Part model, mm, in its own coordinate system. A direction names the side the tool comes from. Give positions to 0.01 mm unless a question says otherwise; leave off trailing zeros. Write each loop counter-clockwise with the first axis right and the second up, starting at its lowest first coordinate (ties: lowest second). Pieces come first, ordered by that corner, then holes. Notation, with made-up numbers: M -34,15.25 L -19,15.25 A17 cw -19,25.25 Z; hole C -23,31 d3. An arc over 180 degrees is marked long. Answer as CSV lines item,"result". Start each with the question number.
1) Tool access for faces 1 (the flat face through (-3, 10, -14.25)), 2 (the cylindrical face through (33.48, 9.6, -12.43)), 3 (the flat face through (-11, 18, -9)): list every direction of +Z, -Z, +X, -X, +Y, -Y with a clear straight run to the whole face (end or side of a thin tool).
2) Mould opens along Z. For faces 4 (the cylindrical face through (33.48, 9.6, 12.43)), 5 (the flat face through (35, 7, 0)), 6 (the flat face through (0, 9, -17.25)) say: pulls with the +Z half, pulls with the -Z half, needs draft (parallel to the pull), parting line crosses it, or undercut.
3) Slice it at A-A, the plane y = 4.5. Give the cut face in (x, z), plus the area to 3 significant figures.
4) Slice it at C-C, the plane y = 15.5. Give the cut face in (x, z), plus the area to 3 significant figures.
5) Slice it at D-D, the plane x = 7. Give the cut face in (y, z), plus the area to 4 significant figures.
6) Slice it at B-B, the plane x = -24. Give the cut face in (y, z).
7) Pin check, flat tips, straight feed: pin 1 Ø1.6 at (x, z) = (-16.5, 10.5) entering from +Y; pin 2 Ø7 at (x, z) = (18.5, 7) entering from +Y. Stop position of each tip, or through.
8) Wall check: line 1 along X through (y, z) = (3.75, 8); line 2 along Z through (x, y) = (17.5, 10); line 3 along X through (y, z) = (14.75, -7). Give the ranges that are in metal, low to high. Write a range as from..to.
```python
from build123d import *

# Parameters (mm, degrees)
SKETCH1_W           = 70
SKETCH1_H           = 34.5
BOSS_EXTRUDE1_DEPTH = 3
SKETCH2_W           = 70
SKETCH2_H           = 34.5
SKETCH2_W_2         = 64
SKETCH2_H_2         = 28.5
EXTRUDE_THIN1_DEPTH = 15
CUT_EXTRUDE1_REACH  = 76.307
SKETCH3_W           = 26
SKETCH3_H           = 5
SKETCH6_W           = 5
SKETCH6_H           = 28.5
BOSS_EXTRUDE2_DEPTH = 15
SKETCH7_W           = 24
SKETCH7_H           = 8.5
BOSS_EXTRUDE3_DEPTH = 15
SKETCH8_W           = 36.5
SKETCH8_H           = 5.5
BOSS_EXTRUDE4_DEPTH = 13.45
FILLET1_R           = 2
FILLET2_R           = 2
CUT_EXTRUDE6_REACH  = 44.972
SKETCH12_W          = 5
SKETCH12_H          = 23.5
SKETCH13_R          = 1.25
CUT_EXTRUDE7_DEPTH  = 10
FILLET4_R           = 2


with BuildPart() as part:
    # Sketch1 → Boss-Extrude1 (new body)
    with BuildSketch(Plane(origin=(0, 0, 0), x_dir=(1, 0, 0), z_dir=(0, 1, 0))):
        Rectangle(SKETCH1_W, SKETCH1_H)
    extrude(amount=BOSS_EXTRUDE1_DEPTH)

    # Sketch2 → Extrude-Thin1 (add)
    with BuildSketch(Plane(origin=(0, 3, 0), x_dir=(1, 0, 0), z_dir=(0, 1, 0))):
        Rectangle(SKETCH2_W, SKETCH2_H)
        Rectangle(SKETCH2_W_2, SKETCH2_H_2, mode=Mode.SUBTRACT)
    extrude(amount=EXTRUDE_THIN1_DEPTH)

    # Sketch3 → Cut-Extrude1 (cut, up to next)
    with BuildSketch(Plane(origin=(35, 0, 0), x_dir=(0, 0, -1), z_dir=(1, 0, 0)), mode=Mode.PRIVATE) as cut_extrude1_sk1:
        with Locations((0, 11.5)):
            Rectangle(SKETCH3_W, SKETCH3_H)
    cut_extrude1_tool1 = extrude(cut_extrude1_sk1.sketch, amount=-CUT_EXTRUDE1_REACH, mode=Mode.PRIVATE) & part.part
    add(cut_extrude1_tool1.solids().sort_by_distance((35, 11.5, 0))[0], mode=Mode.SUBTRACT)

    # Sketch6 → Boss-Extrude2 (add)
    with BuildSketch(Plane(origin=(0, 3, 0), x_dir=(1, 0, 0), z_dir=(0, 1, 0))):
        with Locations((7, 0)):
            Rectangle(SKETCH6_W, SKETCH6_H)
    extrude(amount=BOSS_EXTRUDE2_DEPTH)

    # Sketch7 → Boss-Extrude3 (add)
    with BuildSketch(Plane(origin=(0, 3, 0), x_dir=(1, 0, 0), z_dir=(0, 1, 0))):
        with Locations((-20, 10)):
            Rectangle(SKETCH7_W, SKETCH7_H)
    extrude(amount=BOSS_EXTRUDE3_DEPTH)

    # Sketch8 → Boss-Extrude4 (add)
    with BuildSketch(Plane(origin=(0, 3, 0), x_dir=(1, 0, 0), z_dir=(0, 1, 0))):
        with Locations((-13.75, -11.5)):
            Rectangle(SKETCH8_W, SKETCH8_H)
    extrude(amount=BOSS_EXTRUDE4_DEPTH)

    # Fillet1
    fillet1_edges = [part.edges().sort_by_distance(p)[0] for p in [
        (33.5, 9, 13),
        (33.5, 14, 13),
        (33.5, 14, -13),
        (33.5, 9, -13),
    ]]
    fillet(fillet1_edges, radius=FILLET1_R)

    # Fillet2
    fillet2_edges = [part.edges().sort_by_distance(p)[0] for p in [
        (35, 9, 17.25),
        (-35, 9, 17.25),
        (-35, 9, -17.25),
        (35, 9, -17.25),
    ]]
    fillet(fillet2_edges, radius=FILLET2_R)

    # Cut-Extrude6: up to this face of the body (flat: up to its plane)
    cut_extrude6_end = Plane(part.part.faces().sort_by_distance((33.5, 9, 0))[0])
    # Sketch12 → Cut-Extrude6 (cut, up to the picked face)
    with BuildSketch(Plane(origin=(0, 18, 0), x_dir=(1, 0, 0), z_dir=(0, 1, 0)), mode=Mode.PRIVATE) as cut_extrude6_sk1:
        with Locations((7, 0)):
            Rectangle(SKETCH12_W, SKETCH12_H)
    cut_extrude6_tool1 = split(extrude(cut_extrude6_sk1.sketch, amount=-CUT_EXTRUDE6_REACH, mode=Mode.PRIVATE), bisect_by=cut_extrude6_end, keep=Keep.BOTH, mode=Mode.PRIVATE)
    add(cut_extrude6_tool1.solids().sort_by(Axis((7, 18, 0), (0, -1, 0)))[0], mode=Mode.SUBTRACT)

    # Sketch13 → Cut-Extrude7 (cut)
    with BuildSketch(Plane(origin=(0, 18, 0), x_dir=(1, 0, 0), z_dir=(0, 1, 0))):
        with Locations(Location((7, 14.25, 0), (0, 0, 270))):
            Circle(SKETCH13_R)
        with Locations(Location((7, -14.25, 0), (0, 0, 90))):
            Circle(SKETCH13_R)
    extrude(amount=-CUT_EXTRUDE7_DEPTH, mode=Mode.SUBTRACT)

    # Fillet4
    fillet4_edges = [part.edges().sort_by_distance(p)[0] for p in [
        (4.5, 10.5, -14.25),
    ]]
    fillet(fillet4_edges, radius=FILLET4_R)


solid = part.part
```
Found:
1,face 1,"+Y"
1,face 2,"+X"
1,face 3,"+Z, -Z, +X, -X, +Y"
2,face 4,"undercut"
2,face 5,"needs draft"
2,face 6,"pulls with the -Z half"
3,outline,"M -35,-15.25 A2 ccw -33,-17.25 L 33,-17.25 A2 ccw 35,-15.25 L 35,15.25 A2 ccw 33,17.25 L -33,17.25 A2 ccw -35,15.25 Z; hole M -32,-5.75 L -8,-5.75 L -8,-14.25 L 2.5,-14.25 A2 ccw 4.5,-12.25 L 4.5,8.75 L -32,8.75 Z; hole M 9.5,-14.25 L 32,-14.25 L 32,14.25 L 9.5,14.25 Z"
3,area,"1,140 mm²"
4,outline,"M -35,-15.25 A2 ccw -33,-17.25 L 33,-17.25 A2 ccw 35,-15.25 L 35,15.25 A2 ccw 33,17.25 L -33,17.25 A2 ccw -35,15.25 Z; hole M -32,-5.75 L -8,-5.75 L -8,-14.25 L 2.5,-14.25 A2 ccw 4.5,-12.25 L 4.5,-11.75 L 9.5,-11.75 L 9.5,-14.25 L 32,-14.25 L 32,14.25 L 9.5,14.25 L 9.5,11.75 L 4.5,11.75 L 4.5,8.75 L -32,8.75 Z; hole C 7,-14.25 d2.5; hole C 7,14.25 d2.5"
4,area,"1,010 mm²"
5,outline,"M 0,-17.25 L 18,-17.25 L 18,-15.5 L 8,-15.5 L 8,-13 L 18,-13 L 18,-11.75 L 9,-11.75 L 9,11.75 L 18,11.75 L 18,13 L 8,13 L 8,15.5 L 18,15.5 L 18,17.25 L 0,17.25 Z"
5,area,"359.5 mm²"
6,outline,"M 0,-17.25 L 18,-17.25 L 18,-5.75 L 3,-5.75 L 3,8.75 L 16.45,8.75 L 16.45,14.25 L 18,14.25 L 18,17.25 L 0,17.25 Z"
7,pin 1,"y = 16.45"
7,pin 2,"y = 3"
8,line 1,"-35..-32, 4.5..9.5, 32..35"
8,line 2,"-17.25..-14.25, 14.25..17.25"
8,line 3,"-35..-8, 32..35"
